from build123d import *

# Parameters (mm, degrees)
BODY_DEPTH      = 21
SKETCH2_R       = 1
BOLT_HOLE_DEPTH = 22
EDGE_FILLETS_R  = 1


with BuildPart() as part:
    # Sketch1 → body (new body)
    with BuildSketch(Plane(origin=(0, 0, 0), x_dir=(0, 0, -1), z_dir=(1, 0, 0))):
        Polygon((0, 0), (10, 0), (0, -10), align=None)
    extrude(amount=BODY_DEPTH)

    # Sketch2 → bolt_hole (cut, through all)
    with BuildSketch(Plane.ZY):
        with Locations((-3, -3)):
            Circle(SKETCH2_R)
    extrude(amount=-BOLT_HOLE_DEPTH, mode=Mode.SUBTRACT)

    # edge_fillets
    edge_fillets_edges = [part.edges().sort_by_distance(p)[0] for p in [
        (21, -5, 0),
        (21, -5, -5),
        (0, -5, -5),
        (0, -5, 0),
        (0, 0, -5),
        (21, 0, -5),
        (10.5, 0, -10),
        (10.5, -10, 0),
        (10.5, 0, 0),
    ]]
    fillet(edge_fillets_edges, radius=EDGE_FILLETS_R)


solid = part.part
Source: CAD feature listing. Evaluate the final solid. Frame: model axes, mm. Coordinates: 2 decimals unless noted, no trailing zeros. Order: outer loops, then holes, each group sorted by start corner. A loop starts at its lowest first (then second) coordinate and runs counter-clockwise, first axis right, second up.
Item 1: Cut plane A-A (x = 7). Return loops of the section in (y, z).
Output values:
outline: (-8.29, -1.71) - (-1.71, -8.29) arc R1 ccw to (0, -7.59) - (0, -1) arc R1 ccw to (-1, 0) - (-7.59, 0) arc R1 ccw to start; hole circle Ø2 at (-3, -3)
Item 2: Material intervals for line 1 (Y direction, x = 13, z = -3); line 2 (Y direction, x = 1.5, z = -3.75), sorted ascending.
Output values:
line 1: y = -7 to -4, -2 to 0
line 2: y = -6.25 to -3.66, -2.34 to 0
Item 3: First-contact query: P1, Ø1, axis at x = 6, z = -4, coming from the -Y side; P2, Ø2, axis at x = 11, y = -5.5, coming from the -Z side. Flat tips, straight axial feed; report the tip coordinate or a pass-through.
Output values:
P1: stops at y = -6.5
P2: stops at z = -5.5
Item 4: Pull-direction query (Z, two-part tool) for faces 1 (the face through (20.699, -4.247, -0.285)), 2 (the face through (10.4, -3.6, -3.8)), 3 (the face through (20.699, -0.285, -4.339)); classes: pulls with the +Z half, pulls with the -Z half, needs draft (parallel to the pull), parting line crosses it, or undercut.
Output values:
face 1: pulls with the +Z half
face 2: undercut
face 3: needs draft
